Could you check a few things on this drawing? It's one solid part, dimensions in mm from its lowest x, y, z. A direction names the side the tool comes from. Round coordinates to 2 decimals unless told otherwise and drop trailing zeros. Loops run counter-clockwise (first coordinate to the right, second up) from the corner with the lowest first, then second, coordinate; pieces in that order, holes last. Notation, with made-up numbers: M 35.25,18.25 L 74.25,18.25 A25 cw 74.25,35.25 Z; hole C -30,61.5 d9. An arc over 180 degrees is marked long. Return JSON: item names as keys, results as strings.
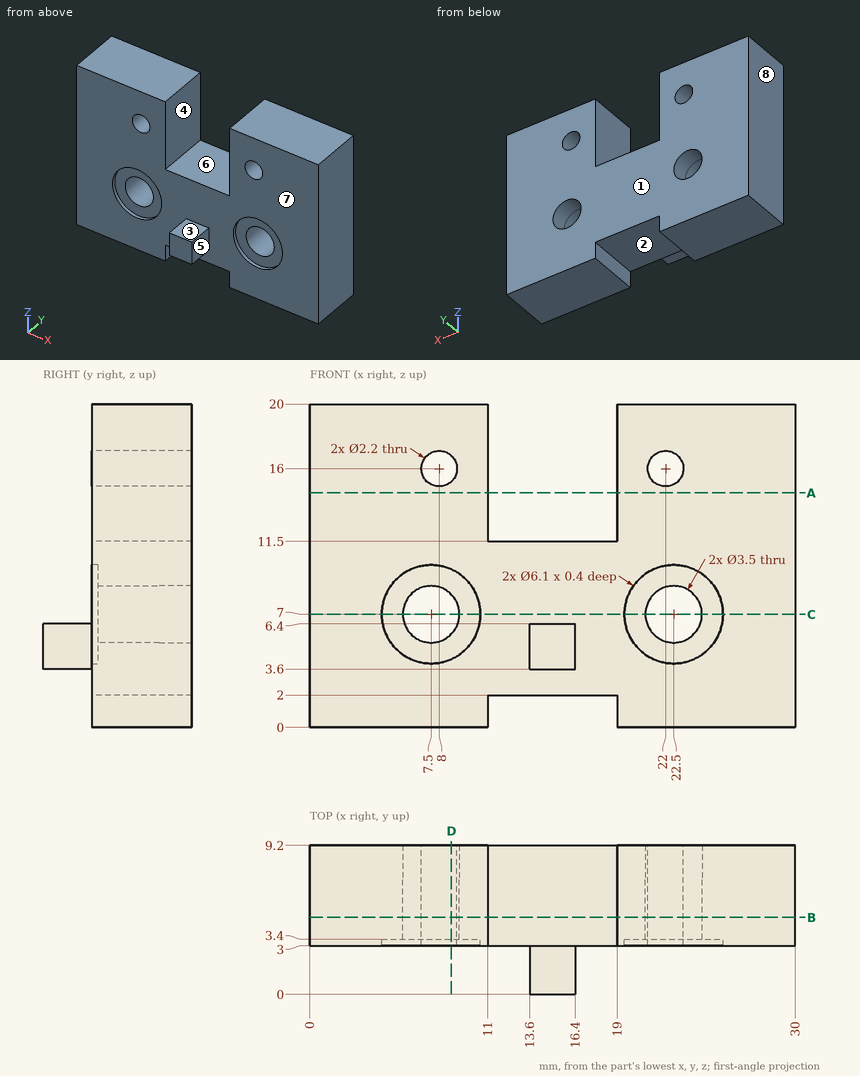
Q1. I'm going to push flat-ended pins straight in: pin 1 Ø2 at (x, z) = (7.5, 7) entering from +Y; pin 2 Ø4 at (x, y) = (12, 2) entering from -Z; pin 3 Ø0.8 at (x, y) = (15, 1) entering from +Z; pin 4 Ø5 at (x, z) = (21, 7.5) entering from -Y. Where does each tip first touch, or does it pass through?
Results:
{"pin 1": "passes through", "pin 2": "stops at z = 0", "pin 3": "stops at z = 6.4", "pin 4": "stops at y = 3"}
Q2. Suppose I cut it at C-C, the plane z = 7. Please give me the cut outline in (x, y).
Results:
{"outline": "M 0,3 L 4.45,3 L 4.45,3.4 L 5.75,3.4 L 5.75,9.2 L 0,9.2 Z; M 9.25,3.4 L 10.55,3.4 L 10.55,3 L 19.45,3 L 19.45,3.4 L 20.75,3.4 L 20.75,9.2 L 9.25,9.2 Z; M 24.25,3.4 L 25.55,3.4 L 25.55,3 L 30,3 L 30,9.2 L 24.25,9.2 Z"}
Q3. On a 3-axis mill with a long thin cutter (end or side, diameter ignored), from which of +Z, -Z, +X, -X, +Y, -Y can I reach the whole of each face in a straight line? I mean the marked faces 1, 2, 3 and 4. Say none if no direction works.
Results:
{"face 1": "+Z, -Z, +X, -X, +Y", "face 2": "-Z, +Y, -Y", "face 3": "+Z, +X, -X, -Y", "face 4": "+Z, +Y, -Y"}
Q4. If I drill on line 1 along X through (y, z) = (8.75, 7); line 2 along X through (y, z) = (6.5, 1.25); line 3 along Z through (x, y) = (22, 7.75), over which ranges is the centre line in solid material (lowest first)?
Results:
{"line 1": "x = 0 to 5.75, 9.25 to 20.75, 24.25 to 30", "line 2": "x = 0 to 11, 19 to 30", "line 3": "z = 0 to 5.32, 8.68 to 14.9, 17.1 to 20"}
Q5. Suppose I cut it at B-B, the plane y = 4.75. Please give me the cut outline in (x, z).
Results:
{"outline": "M 0,0 L 11,0 L 11,2 L 19,2 L 19,0 L 30,0 L 30,20 L 19,20 L 19,11.5 L 11,11.5 L 11,20 L 0,20 Z; hole C 7.5,7 d3.5; hole C 8,16 d2.2; hole C 22.5,7 d3.5; hole C 22,16 d2.2"}
Q6. Suppose I cut it at D-D, the plane x = 8.75. Please give me the cut outline in (y, z), plus the area to 3 significant figures.
Results:
{"outline": "M 3,0 L 9.2,0 L 9.2,5.78 L 3.4,5.78 L 3.4,4.22 L 3,4.22 Z; M 3,9.78 L 3.4,9.78 L 3.4,8.22 L 9.2,8.22 L 9.2,15.2 L 3,15.2 Z; M 3,16.8 L 9.2,16.8 L 9.2,20 L 3,20 Z", "area": "97.6 mm2"}
Q7. Suppose I cut it at A-A, the plane z = 14.5. Please give me the cut outline in (x, y), plus the area to 3 significant figures.
Results:
{"outline": "M 0,3 L 11,3 L 11,9.2 L 0,9.2 Z; M 19,3 L 30,3 L 30,9.2 L 19,9.2 Z", "area": "136 mm2"}
Q8. Thinking about a two-plate mould opening in X: for the marked faces 5, 6, 7 and 8, which applies, pulls with the +X half, pulls with the -X half, needs draft (parallel to the pull), parting line crosses it, or undercut?
Results:
{"face 5": "pulls with the +X half", "face 6": "undercut", "face 7": "needs draft", "face 8": "pulls with the -X half"}
